Input: part model. Units: mm. Frame: model coordinates. Face numbers are marked on the shaded views. A direction names the side the tool comes from. Round coordinates to 2 decimals unless told otherwise and drop trailing zeros. Order: outer loops, then holes, each group sorted by start corner. A loop starts at its lowest first (then second) coordinate and runs counter-clockwise, first axis right, second up.
Item 1: Line query: L1, parallel to X at y = 12, z = 1.15; L2, parallel to Z at x = 10, y = 6. Output: solid intervals per line, ascending.
Item 2: Mould query, pull axis Y, two halves, no side actions, for the marked faces 1, 2 and 3. Classes: released by +Y, released by -Y, zero draft, split by the parting line, or undercut.
Item 3: Cut plane D-D on z = 17.5. Output: boundary loops of the cut face in (x, y), then the cut area to 3 significant figures.
Item 4: Cut plane C-C on x = 2.5. Output: boundary loops of the cut face in (y, z).
Item 5: First-contact query: pin 1 (3 mm diameter, centred on x = 11.03, y = 12, fed in from +Z); pin 2 (5 mm diameter, centred on x = -3.5, y = 8.5, fed in from +Z); pin 3 (6.5 mm diameter, centred on x = -6.47, z = 12, fed in from +Y); pin 4 (4 mm diameter, centred on x = -8.5, z = 9.5, fed in from +Y). Flat tips, straight axial feed; report the tip coordinate or a pass-through.
Item 6: Reachability of the marked faces 4 and 5 from +Z, -Z, +X, -X, +Y, -Y: full face, straight path, thin tool, end or side. Return the list, or none.
Item 7: Cut plane A-A on y = 12. Output: boundary loops of the cut face in (x, z), then the cut area to 4 significant figures.
```python
from build123d import *

# Parameters (mm, degrees)
F0_W                 = 35
F0_H                 = 20
F1_DEPTH             = 4
F2_W                 = 35
F2_H                 = 4
F3_DEPTH             = 16
F6_D                 = 4
F6_CSINK_D           = 7
F6_CSINK_ANGLE       = 90
F6_ON_F4_D           = 4
F6_ON_F4_CSINK_D     = 7
F6_ON_F4_CSINK_ANGLE = 90


with BuildPart() as f1:
    # F0 (on Top) → F1 (new body)
    with BuildSketch(Plane.XY):
        with Locations((2.2826059621, 10)):
            Rectangle(F0_W, F0_H)
    extrude(amount=F1_DEPTH)

    # F2 (on face) → F3 (join)
    with BuildSketch(Plane.XY.offset(4)):
        with Locations((2.2826059621, 2)):
            Rectangle(F2_W, F2_H)
    extrude(amount=F3_DEPTH)

    # F6 (through all)
    with Locations(Plane.XY.offset(4)):
        with Locations((11.0326059621, 12), (-6.4673940379, 12)):
            CounterSinkHole(F6_D / 2, F6_CSINK_D / 2, counter_sink_angle=F6_CSINK_ANGLE)

    # F6 on F4 (through all)
    with Locations(Plane(origin=(0, 4, 0), x_dir=(-1, 0, 0), z_dir=(0, 1, 0))):
        with Locations((6.4673940379, 12), (-11.0326059621, 12)):
            CounterSinkHole(F6_ON_F4_D / 2, F6_ON_F4_CSINK_D / 2, counter_sink_angle=F6_ON_F4_CSINK_ANGLE)


solid = f1.part
```
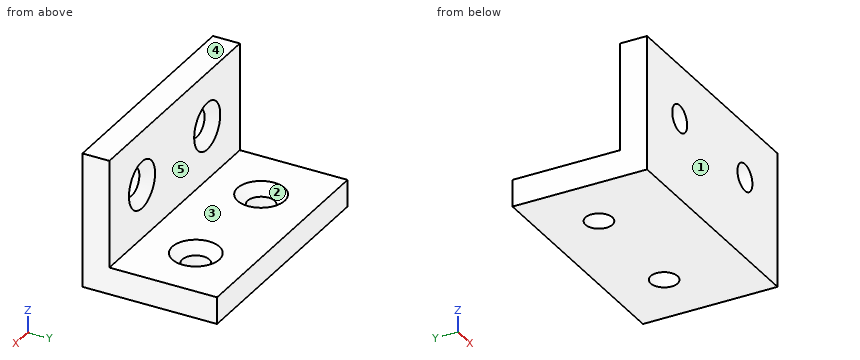
From the geometry:
1. L1: x = -15.22 to -8.47, -4.47 to 9.03, 13.03 to 19.78
1. L2: z = 0 to 4
2. face 1: released by -Y
2. face 2: undercut
2. face 3: zero draft
3. outline: (-15.22, 0) - (19.78, 0) - (19.78, 4) - (-15.22, 4) - close
3. area: 140 mm2
4. outline: (0, 0) - (20, 0) - (20, 4) - (4, 4) - (4, 20) - (0, 20) - close
5. pin 1: passes through
5. pin 2: stops at z = 4
5. pin 3: stops at y = 3.75
5. pin 4: stops at y = 4
6. face 4: +Z, +X, -X, +Y, -Y
6. face 5: +Z, +X, -X, +Y
7. outline: (-15.22, 0) - (-8.47, 0) - (-8.47, 2.5) - (-9.97, 4) - (-15.22, 4) - close; (-4.47, 0) - (9.03, 0) - (9.03, 2.5) - (7.53, 4) - (-2.97, 4) - (-4.47, 2.5) - close; (13.03, 0) - (19.78, 0) - (19.78, 4) - (14.53, 4) - (13.03, 2.5) - close
7. area: 103.5 mm2
